Design review of the part built by this model. Coordinates are the model's own, in mm. A direction names the side the tool comes from. Give positions to 0.01 mm unless a question says otherwise; leave off trailing zeros. Write each loop counter-clockwise with the first axis right and the second up, starting at its lowest first coordinate (ties: lowest second). Pieces come first, ordered by that corner, then holes. Notation, with made-up numbers: (-31.5, 44) -> (22.5, 44) arc R10 cw to (22.5, 57) -> close; hole circle Ø10 at (-27, 31.25). An arc over 180 degrees is marked (long way). Write each question's results on one line, items separated by ' | '. Start each with the question number.
(1) Mouldability with a two-part tool opening along X and no side actions: class faces 1 (the face through (12.7, 38, 5)), 2 (the face through (0, 38, 11.112)), 3 (the face through (11.917, 33.875, -2.198)) as released by +X, released by -X, zero draft, split by the parting line, or undercut.
(2) Take a section at D-D (z = -7). State the section outline as (x, y) points.
(3) To check wall thickness, follow probe 1 along Z at (x, y) = (2, 41); probe 2 along Y at (x, z) = (12.15, 0). State the ranges of each line that lie inside material, in increasing order.
(4) For faces 4 (the face through (11.3, 0, 0.1)), 5 (the face through (11.112, 38, 5)), list the 3-axis set-ups (+Z, -Z, +X, -X, +Y, -Y) from which the entire face can be reached by the end or side of a thin tool; tool diameter is ignored.
(5) Take a section at A-A (y = 22). State the section outline as (x, z) points, plus the area to 3 significant figures.
(6) Take a section at B-B (z = 0). State the section outline as (x, y) points.
(7) Take a section at C-C (x = 4). State the section outline as (y, z) points.
Autodesk Inventor part; units mm, degrees
ref_plane "YZ Plane" through (0, 0, 0) normal (1, 0, 0) x (0, 1, 0)
ref_plane "XZ Plane" through (0, 0, 0) normal (0, 1, 0) x (-1, 0, 0)
ref_plane "XY Plane" through (0, 0, 0) normal (0, 0, 1) x (1, 0, 0)
sketch "Sketch1" plane through (0, 0, 0) normal (0, 1, 0) x (-1, 0, 0)
  line L0 (12.7, 12.7) -> (12.7, -12.7)
  line L1 (12.7, -12.7) -> (-12.7, -12.7)
  line L2 (-12.7, -12.7) -> (-12.7, 12.7)
  line L3 (-12.7, 12.7) -> (12.7, 12.7)
  line L4 (12.7, 12.7) -> (-12.7, -12.7) construction
  line L5 (12.7, -12.7) -> (-12.7, 12.7) construction
  line L6 (11.1125, 11.1125) -> (11.1125, -11.1125)
  line L7 (11.1125, -11.1125) -> (-11.1125, -11.1125)
  line L8 (-11.1125, -11.1125) -> (-11.1125, 11.1125)
  line L9 (-11.1125, 11.1125) -> (11.1125, 11.1125)
  line L10 (11.1125, 11.1125) -> (-11.1125, -11.1125) construction
  line L11 (11.1125, -11.1125) -> (-11.1125, 11.1125) construction
  point P0 (0, 0)
  dimension "d0" = 25.4
  dimension "d1" = 25.4
  dimension "d2" = 1.5875
  dimension "d3" = 1.5875
extrude "Extrusion1" add sketch "Sketch1" along normal blind 660.4
sketch "Sketch2" plane through (12.7, 0, 12.7) normal (1, 0, 0) x (0, 0, -1)
  line L0 (12.7, 0) -> (12.7, 38.1)
  circle A0 centre (12.7, 38.1) radius 4.7625
  line L1 (3.9688, 38.1) -> (8.3344, 45.6615)
  line L2 (8.3344, 45.6615) -> (17.0656, 45.6615)
  line L3 (17.0656, 45.6615) -> (21.4313, 38.1)
  line L4 (21.4313, 38.1) -> (17.0656, 30.5385)
  line L5 (17.0656, 30.5385) -> (8.3344, 30.5385)
  line L6 (8.3344, 30.5385) -> (3.9688, 38.1)
  dimension "d6" = 38.1
  dimension "d7" = 9.525
  dimension "d8" = 8.7312
extrude "Extrusion2" cut sketch "Sketch2" against normal blind 46.6 contours A0
sketch "Sketch3" plane through (12.7, 0, 12.7) normal (1, 0, 0) x (0, 0, -1)
  line L0 (12.7, 0) -> (12.7, 177.8)
  line L1 (0, 0) -> (0, 660.4)
  line L2 (0, 177.8) -> (180.4268, 177.8)
  line L3 (180.4268, 177.8) -> (180.4268, 742.2297)
  line L4 (180.4268, 742.2297) -> (0, 742.2297)
  line L5 (0, 742.2297) -> (0, 177.8)
  dimension "d11" = 177.8
extrude "Extrusion3" cut sketch "Sketch3" against normal blind 354.85
sketch "Sketch4" plane through (12.7, 0, 12.7) normal (1, 0, 0) x (0, 0, -1)
  point P0 (12.7, 0)
sketch "Sketch5" plane through (12.7, 0, 12.7) normal (1, 0, 0) x (0, 0, -1)
  line L0 (12.7, 0) -> (12.7, 114.3)
  line L1 (12.7, 114.3) -> (91.9102, 114.3)
  line L2 (91.9102, 114.3) -> (43.6603, 200.7395)
  line L3 (43.6603, 200.7395) -> (-39.5707, 207.1728)
  line L4 (-39.5707, 207.1728) -> (-50.6279, 117.9106)
  line L5 (-50.6279, 117.9106) -> (-45.0993, 114.3)
  line L6 (-45.0993, 114.3) -> (12.7, 114.3)
  dimension "d14" = 114.3
extrude "Extrusion4" cut sketch "Sketch5" against normal blind 40.85
sketch "Sketch6" plane through (12.7, 114.3, 12.7) normal (0, 1, 0) x (1, 0, 0)
  line L0 (0, 0) -> (-25.4, 0)
  line L1 (0, 25.4) -> (0, 0)
  line L2 (-25.4, 25.4) -> (0, 25.4)
  line L3 (-25.4, 0) -> (-25.4, 25.4)
  line L4 (-1.5875, 23.8125) -> (-23.8125, 23.8125)
  line L5 (-1.5875, 1.5875) -> (-1.5875, 23.8125)
  line L6 (-23.8125, 1.5875) -> (-1.5875, 1.5875)
  line L7 (-23.8125, 23.8125) -> (-23.8125, 1.5875)
  point P0 (-12.7, 12.7)
extrude "Extrusion5" cut sketch "Sketch6" against normal blind 38.1
properties part number "Tube End" material "Aluminum 6061"
Report:
1) face 1: released by +X | face 2: undercut | face 3: zero draft
2) outline: (-12.7, 0) -> (-11.11, 0) -> (-11.11, 76.2) -> (-12.7, 76.2) -> close; (11.11, 0) -> (12.7, 0) -> (12.7, 76.2) -> (11.11, 76.2) -> close
3) probe 1: -12.7 to -11.11, 11.11 to 12.7 | probe 2: 0 to 33.34, 42.86 to 76.2
4) face 4: +Z, -Z, +X, -X, -Y | face 5: +Y, -Y
5) outline: (-12.7, -12.7) -> (12.7, -12.7) -> (12.7, 12.7) -> (-12.7, 12.7) -> close; hole (-11.11, -11.11) -> (11.11, -11.11) -> (11.11, 11.11) -> (-11.11, 11.11) -> close | area: 151 mm2
6) outline: (-12.7, 0) -> (-11.11, 0) -> (-11.11, 33.34) -> (-12.7, 33.34) -> close; (-12.7, 42.86) -> (-11.11, 42.86) -> (-11.11, 76.2) -> (-12.7, 76.2) -> close; (11.11, 0) -> (12.7, 0) -> (12.7, 33.34) -> (11.11, 33.34) -> close; (11.11, 42.86) -> (12.7, 42.86) -> (12.7, 76.2) -> (11.11, 76.2) -> close
7) outline: (0, -12.7) -> (76.2, -12.7) -> (76.2, -11.11) -> (0, -11.11) -> close; (0, 11.11) -> (76.2, 11.11) -> (76.2, 12.7) -> (0, 12.7) -> close
